Autodesk Inventor part; units mm, degrees
ref_plane "YZ Plane" through (0, 0, 0) normal (1, 0, 0) x (0, 1, 0)
ref_plane "XZ Plane" through (0, 0, 0) normal (0, 1, 0) x (-1, 0, 0)
ref_plane "XY Plane" through (0, 0, 0) normal (0, 0, 1) x (1, 0, 0)
sketch "Sketch1" plane through (0, 0, 0) normal (0, 0, 1) x (1, 0, 0)
  line L0 (-12.7, -25.4) -> (12.7, -25.4)
  line L1 (12.7, -25.4) -> (12.7, 25.4)
  line L2 (12.7, 25.4) -> (-12.7, 25.4)
  line L3 (-12.7, 25.4) -> (-12.7, -25.4)
  line L4 (-12.7, -25.4) -> (12.7, 25.4) construction
  line L5 (12.7, -25.4) -> (-12.7, 25.4) construction
  line L6 (-10.16, -22.86) -> (10.16, -22.86)
  line L7 (10.16, -22.86) -> (10.16, 22.86)
  line L8 (10.16, 22.86) -> (-10.16, 22.86)
  line L9 (-10.16, 22.86) -> (-10.16, -22.86)
  line L10 (-10.16, -22.86) -> (10.16, 22.86) construction
  line L11 (10.16, -22.86) -> (-10.16, 22.86) construction
  point P0 (0, 0)
  dimension "d0" = 25.4
  dimension "d1" = 50.8
  dimension "d2" = 20.32
  dimension "d3" = 45.72
extrude "Extrusion1" add sketch "Sketch1" along normal mid plane 50.8
sketch "Sketch2" plane through (-12.7, 25.4, 25.4) normal (0, 1, 0) x (1, 0, 0)
  line L0 (25.4, 0) -> (0, 0)
  line L1 (25.4, 50.8) -> (25.4, 0)
  point P0 (12.7, 25.4)
  point P1 (12.7, 12.7)
  point P2 (13.5104, 38.1)
  dimension "d6" = 25.4
  dimension "d7" = 12.7
  dimension "d8" = 12.7
hole "Hole1" at (0, 25.4, 12.7) at (0.8104, 25.4, -12.7) direction (0, -1, 0) diameter 4.1402 end through all
sketch "Sketch3" plane through (12.7, -25.4, 25.4) normal (1, 0, 0) x (0, 0, -1)
  point P0 (25.4, 25.4)
  point P1 (25.4, 25.4)
hole "Hole2" at (12.7, 0, 0) direction (-1, 0, 0) diameter 28.5496 end through all
properties part number "Pulley_holder"
Build history of the part. All positions in model axes, mm. A direction names the side the tool comes from. Give positions to 0.01 mm unless a question says otherwise; leave off trailing zeros. Order: outer loops, then holes, each group sorted by start corner. A loop starts at its lowest first (then second) coordinate and runs counter-clockwise, first axis right, second up. Notation, with made-up numbers: M 73.25,-10.5 L 131.25,-10.5 A21 ccw 131.25,2.5 Z; hole C -39,35.25 d10. An arc over 180 degrees is marked long. Use one line per item in the form item = value.
Q1. Wall check: probe 1 along Y at (x, z) = (8.75, -18); probe 2 along X at (y, z) = (11.5, -14); probe 3 along Z at (x, y) = (0, 24). Give the ranges that are in metal, low to high.
Conclusion:
probe_1 = -25.4 to -22.86, 22.86 to 25.4
probe_2 = -12.7 to -10.16, 10.16 to 12.7
probe_3 = -25.4 to -14.6, -10.8 to 10.63, 14.77 to 25.4
Q2. Pull direction X, two halves, no side cores. Call faces 1 (the flat face through (0, -22.86, 0)), 2 (the flat face through (0, 25.4, 0)), 3 (the flat face through (-12.7, -11, 11)): released by +X, released by -X, zero draft, split by the parting line, or undercut.
Conclusion:
face_1 = undercut
face_2 = zero draft
face_3 = released by -X
Q3. Pin check, flat tip, straight feed: P1, Ø2.5, axis at x = 0, z = 12.7, coming from the +Y side. Stop position of the tip, or through.
Conclusion:
P1 = through
Q4. Which spindle directions (+Z, -Z, +X, -X, +Y, -Y) get a long thin tool onto all of the face, cutting with end or side? Do faces 4 (the cylindrical face through (-0.09, -24.15, 10.63)), 5 (the flat face through (0, 22.86, 0)). Say none if no direction does.
Conclusion:
face_4 = +Y, -Y
face_5 = +Z, -Z
Q5. Slice it at B-B, the plane y = 16. Write the cut outline in (x, z).
Conclusion:
outline = M -12.7,-25.4 L -10.16,-25.4 L -10.16,25.4 L -12.7,25.4 Z; M 10.16,-25.4 L 12.7,-25.4 L 12.7,25.4 L 10.16,25.4 Z
Q6. Slice it at C-C, the plane z = 21. Write the cut outline in (x, y), and give its area (3 significant figures).
Conclusion:
outline = M -12.7,-25.4 L 12.7,-25.4 L 12.7,25.4 L -12.7,25.4 Z; hole M -10.16,-22.86 L 10.16,-22.86 L 10.16,22.86 L -10.16,22.86 Z
area = 361 mm2
Q7. Slice it at A-A, the plane x = -5. Write the cut outline in (y, z), and give its area (3 significant figures).
Conclusion:
outline = M -25.4,-25.4 L -22.86,-25.4 L -22.86,25.4 L -25.4,25.4 Z; M 22.86,-25.4 L 25.4,-25.4 L 25.4,25.4 L 22.86,25.4 Z
area = 258 mm2
Q8. Slice it at D-D, the plane z = 2.5. Write the cut outline in (x, y), and give its area (3 significant figures).
Conclusion:
outline = M -12.7,-25.4 L 12.7,-25.4 L 12.7,-14.05 L 10.16,-14.05 L 10.16,-22.86 L -10.16,-22.86 L -10.16,-14.05 L -12.7,-14.05 Z; M -12.7,14.05 L -10.16,14.05 L -10.16,22.86 L 10.16,22.86 L 10.16,14.05 L 12.7,14.05 L 12.7,25.4 L -12.7,25.4 Z
area = 218 mm2
